from build123d import *

# Parameters (mm, degrees)
SKETCH1_W           = 407.9875
SKETCH1_H           = 88.9
BOSS_EXTRUDE1_DEPTH = 38.1
SKETCH3_W           = 88.9
SKETCH3_H           = 38.1
CUT_EXTRUDE2_DEPTH  = 39.1
SKETCH4_W           = 69.85
SKETCH4_H           = 19.05
CUT_EXTRUDE3_DEPTH  = 89.9


with BuildPart() as part:
    # Sketch1 → Boss-Extrude1 (new body)
    with BuildSketch(Plane(origin=(0, 0, 0), x_dir=(1, 0, 0), z_dir=(0, 1, 0))):
        with Locations((203.99375, 44.45)):
            Rectangle(SKETCH1_W, SKETCH1_H)
    extrude(amount=BOSS_EXTRUDE1_DEPTH)

    # Sketch3 → Cut-Extrude2 (cut, through all)
    with BuildSketch(Plane(origin=(0, 38.1, 0), x_dir=(1, 0, 0), z_dir=(0, 1, 0))):
        with Locations((363.5375, 69.85)):
            Rectangle(SKETCH3_W, SKETCH3_H)
    extrude(amount=-CUT_EXTRUDE2_DEPTH, mode=Mode.SUBTRACT)

    # Sketch4 → Cut-Extrude3 (cut, through all)
    with BuildSketch(Plane.XY):
        with Locations((34.925, 9.525)):
            Rectangle(SKETCH4_W, SKETCH4_H)
    extrude(amount=-CUT_EXTRUDE3_DEPTH, mode=Mode.SUBTRACT)


solid = part.part
The listing builds one solid part. Answer for the finished solid, in the listing's coordinates (mm). A direction names the side the tool comes from. Round coordinates to 2 decimals unless told otherwise and drop trailing zeros. Order: outer loops, then holes, each group sorted by start corner. A loop starts at its lowest first (then second) coordinate and runs counter-clockwise, first axis right, second up. Notation, with made-up numbers: (5.5, 82.5) -> (21.5, 82.5) arc R23 cw to (21.5, 100.5) -> close; hole circle Ø3 at (-14.75, -35). An arc over 180 degrees is marked (long way). Write each question's results on one line, items separated by ' | '. Start each with the question number.
Q1. Find section C-C (x = 375.5). Determine the outline of the cut face in (y, z).
Q2. Find section A-A (y = 13.5). Determine the outline of the cut face in (x, z), then the cut area to 3 significant figures.
Q3. Straight lines are drawn through the part: probe 1 along X at (y, z) = (17.5, -74); probe 2 along Y at (x, z) = (21.5, -38.5); probe 3 along X at (y, z) = (22.5, -52.5). For each, find the intervals that lie inside material, in ascending order. Write a range as from..to.
Q4. Which of the six approach directions +Z, -Z, +X, -X, +Y, -Y give full straight-line access (tool end or side, diameter ignored) to faces 1 (the flat face through (34, 19.05, -44)), 2 (the flat face through (157, 19, -88.9)), 3 (the flat face through (319.088, 19, -70))?
Q5. Find section B-B (z = -70). Determine the outline of the cut face in (x, y).
Q6. This flat-tipped pin is pushed along its axis until it touches: pin 1 (3 mm diameter, centred on y = 4.5, z = -26, fed in from -X). Where does it stop, or does it pass through?
Worked answers:
1) outline: (0, -50.8) -> (38.1, -50.8) -> (38.1, 0) -> (0, 0) -> close
2) outline: (69.85, -88.9) -> (319.09, -88.9) -> (319.09, -50.8) -> (407.99, -50.8) -> (407.99, 0) -> (69.85, 0) -> close | area: 26,700 mm2
3) probe 1: x = 69.85..319.09 | probe 2: y = 19.05..38.1 | probe 3: x = 0..319.09
4) face 1: +Z, -Z, -X, -Y | face 2: -Z, +X, -X, +Y, -Y | face 3: -Z, +X, +Y, -Y
5) outline: (0, 19.05) -> (69.85, 19.05) -> (69.85, 0) -> (319.09, 0) -> (319.09, 38.1) -> (0, 38.1) -> close
6) pin 1: stops at x = 69.85
